The drawing under review shows one solid part. Ordinate dimensions are in mm from its lowest x, y, z. Coordinates: 2 decimals unless noted, no trailing zeros. Write each loop counter-clockwise with the first axis right and the second up, starting at its lowest first coordinate (ties: lowest second). Pieces come first, ordered by that corner, then holes.
Q1. The part is to be moulded in two halves that separate along Y. For the marked faces 1, 2 and 3, say which applies: +Y half, -Y half, draft (parallel to the pull), parting line (faces both ways), or undercut.
Q2. Add section A-A, the plane z = 10. Give the number of separate pieces and of enclosed holes in the cut face, plus the area to 3 significant figures.
Q3. Add section C-C, the plane x = 1.25. Give the boundary of the cut face in (y, z) (1 decimal), plus the area to 3 significant figures.
Q4. To check wall thickness, follow probe 1 along Z at (x, y) = (5.5, 22) (1 decimal); probe 2 along Y at (x, z) = (5, 3.5); probe 3 along Y at (x, z) = (0.5, 3) (1 decimal). State the ranges of each line that lie inside material, in increasing order.
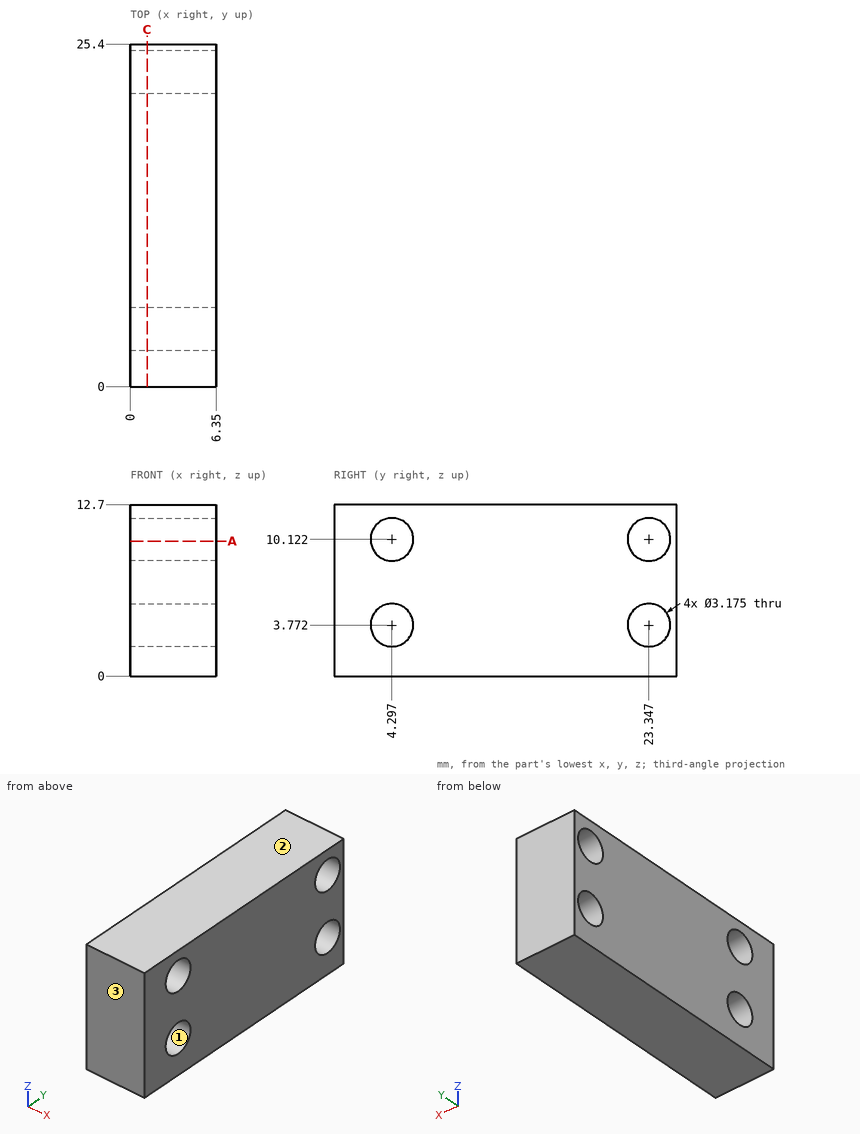
Here are the results:
1. face 1: undercut
1. face 2: draft
1. face 3: -Y half
2. separate pieces: 3
2. enclosed holes: 0
2. area: 121 mm2
3. outline: (0, 0) - (25.4, 0) - (25.4, 12.7) - (0, 12.7) - close; hole circle Ø3.2 at (4.3, 3.8); hole circle Ø3.2 at (4.3, 10.1); hole circle Ø3.2 at (23.3, 3.8); hole circle Ø3.2 at (23.3, 10.1)
3. area: 291 mm2
4. probe 1: z = 0 to 2.9, 4.6 to 9.3, 11 to 12.7
4. probe 2: y = 0 to 2.73, 5.86 to 21.78, 24.91 to 25.4
4. probe 3: y = 0 to 2.9, 5.7 to 22, 24.7 to 25.4
